```python
from build123d import *

# Parameters (mm, degrees)
SKETCH1_W           = 53.964084124
SKETCH1_H           = 13.786930342
SKETCH1_R           = 2
BOSS_EXTRUDE1_DEPTH = 6.4
SKETCH3_R           = 1
BOSS_EXTRUDE2_DEPTH = 6.4
SKETCH4_R           = 4.25
CUT_EXTRUDE1_DEPTH  = 4.5
SKETCH5_W           = 11
SKETCH5_H           = 6
CUT_EXTRUDE2_DEPTH  = 7.4
SKETCH6_W           = 32
SKETCH6_H           = 32
CUT_EXTRUDE3_DEPTH  = 3
FILLET2_R           = 2
FILLET3_R           = 5
CUT_EXTRUDE4_DEPTH  = 3.5
CUT_EXTRUDE5_DEPTH  = 10


with BuildPart() as part:
    # Sketch1 → Boss-Extrude1 (new body)
    with BuildSketch(Plane(origin=(0, 0, 0), x_dir=(1, 0, 0), z_dir=(0, 1, 0))):
        Rectangle(SKETCH1_W, SKETCH1_H)
        with Locations((-19, 0)):
            Circle(SKETCH1_R, mode=Mode.SUBTRACT)
        with Locations((19, 0)):
            Circle(SKETCH1_R, mode=Mode.SUBTRACT)
    extrude(amount=BOSS_EXTRUDE1_DEPTH)

    # Sketch3 → Boss-Extrude2 (add)
    with BuildSketch(Plane(origin=(0, 6.4, 0), x_dir=(1, 0, 0), z_dir=(0, 1, 0))):
        with BuildLine():
            Line((19, 2), (19, 21.5))
            Line((19, 21.5), (-19, 21.5))
            Line((-19, 21.5), (-19, 2))
            ThreePointArc((-19, 2), (-17, 0), (-19, -2))
            Line((-19, -2), (-19, -16.5))
            Line((-19, -16.5), (19, -16.5))
            Line((19, -16.5), (19, -2))
            ThreePointArc((19, -2), (17, 0), (19, 2))
        make_face()
        with Locations((-17, 19.5)):
            Circle(SKETCH3_R, mode=Mode.SUBTRACT)
        with Locations((17, 19.5)):
            Circle(SKETCH3_R, mode=Mode.SUBTRACT)
        with Locations((-17, -14.5)):
            Circle(SKETCH3_R, mode=Mode.SUBTRACT)
        with Locations((17, -14.5)):
            Circle(SKETCH3_R, mode=Mode.SUBTRACT)
    extrude(amount=-BOSS_EXTRUDE2_DEPTH)

    # Sketch4 → Cut-Extrude1 (cut)
    with BuildSketch(Plane(origin=(0, 6.4, 0), x_dir=(1, 0, 0), z_dir=(0, 1, 0))):
        with Locations((-19, 0)):
            Circle(SKETCH4_R)
        with Locations((19, 0)):
            Circle(SKETCH4_R)
    extrude(amount=-CUT_EXTRUDE1_DEPTH, mode=Mode.SUBTRACT)

    # Sketch5 → Cut-Extrude2 (cut, through all)
    with BuildSketch(Plane(origin=(0, 6.4, 0), x_dir=(1, 0, 0), z_dir=(0, 1, 0))):
        with Locations((5, -11)):
            Rectangle(SKETCH5_W, SKETCH5_H)
    extrude(amount=-CUT_EXTRUDE2_DEPTH, mode=Mode.SUBTRACT)

    # Sketch6 → Cut-Extrude3 (cut)
    with BuildSketch(Plane(origin=(0, 6.4, 0), x_dir=(1, 0, 0), z_dir=(0, 1, 0))):
        with Locations((0, 2.5)):
            Rectangle(SKETCH6_W, SKETCH6_H)
    extrude(amount=-CUT_EXTRUDE3_DEPTH, mode=Mode.SUBTRACT)

    # Fillet2
    fillet2_edges = [part.edges().sort_by_distance(p)[0] for p in [
        (-19, 3.2, 16.5),
        (19, 3.2, -21.5),
        (-19, 3.2, -21.5),
        (19, 3.2, -6.893465171),
        (19, 3.2, 6.893465171),
        (19, 3.2, 16.5),
        (-19, 3.2, 6.893465171),
        (-19, 3.2, -6.893465171),
        (26.982042062, 3.2, 6.893465171),
        (-26.982042062, 3.2, 6.893465171),
        (-26.982042062, 3.2, -6.893465171),
        (26.982042062, 3.2, -6.893465171),
    ]]
    fillet(fillet2_edges, radius=FILLET2_R)

    # Fillet3
    fillet3_edges = [part.edges().sort_by_distance(p)[0] for p in [
        (16, 4.9, -18.5),
        (-16, 4.9, 13.5),
        (16, 4.9, 13.5),
        (-16, 4.9, -18.5),
    ]]
    fillet(fillet3_edges, radius=FILLET3_R)

    # Sketch7 → Cut-Extrude4 (cut)
    with BuildSketch(Plane.XZ):
        with BuildLine():
            Line((-17, -17.5), (-19, -17.5))
            Line((-19, -17.5), (-19, -21.5))
            Line((-19, -21.5), (-15, -21.5))
            Line((-15, -21.5), (-15, -19.5))
            ThreePointArc((-15, -19.5), (-15.585786438, -18.085786438), (-17, -17.5))
        make_face()
        with BuildLine():
            Line((15, -19.5), (15, -21.5))
            Line((15, -21.5), (19, -21.5))
            Line((19, -21.5), (19, -17.5))
            Line((19, -17.5), (17, -17.5))
            ThreePointArc((17, -17.5), (15.585786438, -18.085786438), (15, -19.5))
        make_face()
        with BuildLine():
            Line((-17, 12.5), (-19, 12.5))
            Line((-19, 12.5), (-19, 16.5))
            Line((-19, 16.5), (-15, 16.5))
            Line((-15, 16.5), (-15, 14.5))
            ThreePointArc((-15, 14.5), (-15.585786438, 13.085786438), (-17, 12.5))
        make_face()
        with BuildLine():
            Line((17, 12.5), (19, 12.5))
            Line((19, 12.5), (19, 16.5))
            Line((19, 16.5), (15, 16.5))
            Line((15, 16.5), (15, 14.5))
            ThreePointArc((15, 14.5), (15.585786438, 13.085786438), (17, 12.5))
        make_face()
    extrude(amount=-CUT_EXTRUDE4_DEPTH, mode=Mode.SUBTRACT)

    # Sketch8 → Cut-Extrude5 (cut, symmetric)
    with BuildSketch(Plane(origin=(0, 0, 0), x_dir=(0, 0, -1), z_dir=(1, 0, 0))):
        Polygon((-10, 0), (-16.5, 6), (-16.5, 0), align=None)
    extrude(amount=CUT_EXTRUDE5_DEPTH, both=True, mode=Mode.SUBTRACT)


solid = part.part
```
Input: part model. Units: mm. Frame: model coordinates. A direction names the side the tool comes from. Round coordinates to 2 decimals unless told otherwise and drop trailing zeros. Loops run counter-clockwise (first coordinate to the right, second up) from the corner with the lowest first, then second, coordinate; pieces in that order, holes last. Notation, with made-up numbers: (24.5, 7.5) -> (59.5, 7.5) arc R23 ccw to (59.5, 32.5) -> close; hole circle Ø8 at (28.25, 0.25). An arc over 180 degrees is marked (long way). One line per item, written item: value.
(1) Set-up query: faces 5 (the face through (18, 2, 12.5)), 6 (the face through (-19, 3, -14)), 7 (the face through (23, 3, 6.893)), 8 (the face through (17.9, 3.5, -20.4)). Return all of +Z, -Z, +X, -X, +Y, -Y with unobstructed straight access to the full face (end or side cutting, diameter ignored); none if empty.
Geometry check:
face 5: +Z, +X, -Y
face 6: -Z, -X, +Y, -Y
face 7: +Z, +X, +Y, -Y
face 8: -Z, +X, -Y
(2) Mould query, pull axis Z, two halves, no side actions, for faces 1 (the face through (18.4, 4.93, 15.93)), 2 (the face through (-15, 2, -21)), 3 (the face through (-16.54, 4.97, -18.61)), 4 (the face through (26.381, 3.245, -6.323)). Classes: pulls with the +Z half, pulls with the -Z half, needs draft (parallel to the pull), parting line crosses it, or undercut.
Geometry check:
face 1: pulls with the +Z half
face 2: needs draft
face 3: undercut
face 4: pulls with the -Z half
(3) Section C-C (z = -6). Return the cut outline in (x, y).
Geometry check:
outline: (-26.65, 0) -> (26.65, 0) -> (26.65, 6.4) -> (16, 6.4) -> (16, 3.4) -> (-16, 3.4) -> (-16, 6.4) -> (-26.65, 6.4) -> close
(4) Section D-D (x = -14). Return the cut outline in (y, z).
Geometry check:
outline: (0, -21.5) -> (6.4, -21.5) -> (6.4, -17.5) -> (3.4, -17.5) -> (3.4, 12.5) -> (6.4, 12.5) -> (6.4, 16.5) -> (0, 16.5) -> close
(5) Material intervals for line 1 (X direction, y = 0.9, z = 0); line 2 (X direction, y = 4.2, z = 14.5); line 3 (X direction, y = 3.8, z = 0), sorted ascending. Write a range as [from, to].
Geometry check:
line 1: [-26.98, -21], [-17, 17], [21, 26.98]
line 2: [-19, -18], [-16, 16], [18, 19]
line 3: [-26.98, -23.25], [23.25, 26.98]
(6) Pin query (flat end, axial travel): pin 1 (3 mm diameter, centred on x = 16, z = 14, fed in from -Y); pin 2 (3 mm diameter, centred on x = -17.5, z = -19.5, fed in from -Y); pin 3 (2 mm diameter, centred on x = 18, y = 2, fed in from -Z); pin 4 (0.9 mm diameter, centred on y = 5.5, z = 6.5, fed in from -X). Return the tip coordinate at first contact, or that it passes through.
Geometry check:
pin 1: y = 0
pin 2: y = 3.5
pin 3: z = -17.5
pin 4: x = -26.61
(7) Section B-B (x = 9). Return the cut outline in (y, z), plus the area to 3 significant figures.
Geometry check:
outline: (0, -21.5) -> (6.4, -21.5) -> (6.4, -18.5) -> (3.4, -18.5) -> (3.4, 8) -> (0, 8) -> close; (3.69, 14) -> (6.4, 14) -> (6.4, 16.5) -> (6, 16.5) -> close
area: 113 mm2
(8) Section A-A (x = -6). Return the cut outline in (y, z).
Geometry check:
outline: (0, -21.5) -> (6.4, -21.5) -> (6.4, -18.5) -> (3.4, -18.5) -> (3.4, 13.5) -> (6.4, 13.5) -> (6.4, 16.5) -> (6, 16.5) -> (0, 10) -> close
